```python
from build123d import *

# Parameters (mm, degrees)
F0_R      = 57.15
F3_DEPTH  = 514.096
F2_R      = 57.15
F5_DEPTH  = 104.648
F6_W      = 58.42
F6_H      = 58.42
F7_DEPTH  = 58.42
F8_W      = 58.42
F8_H      = 58.42
F9_DEPTH  = 58.42
F10_W     = 44.45
F10_H     = 44.45
F11_DEPTH = 30.48


# Not quite as in the source:
# - a feature names something its author has since deleted; it is built from what else it names


with BuildPart() as f3:
    # F0 (on Right) → F3 (new body)
    with BuildSketch(Plane.YZ):
        Circle(F0_R)
    extrude(amount=F3_DEPTH)

    # F1 (on Top) → F4 (revolve)
    with BuildSketch(Plane.XY):
        with BuildLine():
            Line((514.096, 57.15), (514.096, 0))
            Line((514.096, 0), (615.696, 0))
            Line((615.696, 0), (615.696, 44.45))
            add(Edge.make_bspline(
                [(514.096, 57.15), (530.3059150596, 55.8042351211), (558.1923144484, 54.3135523686), (580.3852464856, 48.6501982027), (594.1085406783, 43.9680323111), (608.3163207178, 44.8236773325), (615.696, 44.45)],
                knots=[0, 0, 0, 0, 0.3407026007, 0.5771106283, 0.7657914869, 1, 1, 1, 1], degree=3))
        make_face()
    revolve(axis=Axis((564.896, 0, 0), (-1, 0, 0)))

    # F2 (on Front) → F5 (join)
    with BuildSketch(Plane.XZ):
        with Locations((257.048, 0)):
            Circle(F2_R)
    extrude(amount=F5_DEPTH)

    # F6 (on face) → F7 (cut)
    with BuildSketch(Plane(origin=(0, 0, 0), x_dir=(0, -1, 0), z_dir=(-1, 0, 0))):
        Rectangle(F6_W, F6_H)
    extrude(amount=-F7_DEPTH, mode=Mode.SUBTRACT)

    # F8 (on face) → F9 (cut)
    with BuildSketch(Plane.XZ.offset(104.648)):
        with Locations((257.048, 0)):
            Rectangle(F8_W, F8_H)
    extrude(amount=-F9_DEPTH, mode=Mode.SUBTRACT)

    # F10 (on face) → F11 (cut)
    with BuildSketch(Plane.YZ.offset(615.696)):
        Rectangle(F10_W, F10_H)
    extrude(amount=-F11_DEPTH, mode=Mode.SUBTRACT)


solid = f3.part
```
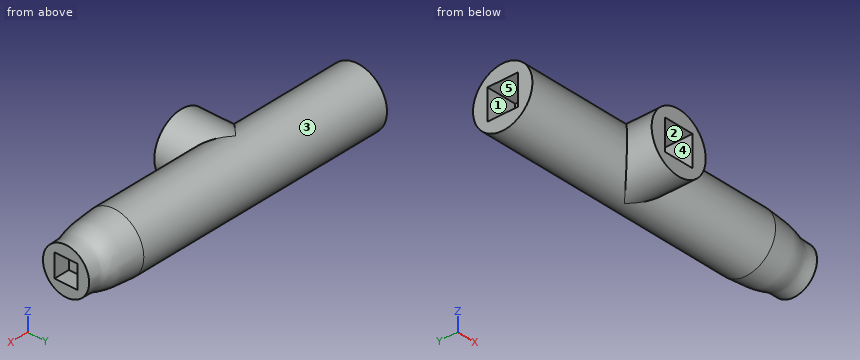
Work out the finished part from the listing and answer in its coordinate system (mm). Face numbers are marked on the shaded views. A direction names the side the tool comes from. Round coordinates to 2 decimals unless told otherwise and drop trailing zeros. Loops run counter-clockwise (first coordinate to the right, second up) from the corner with the lowest first, then second, coordinate; pieces in that order, holes last.
(1) The part is cut by section A-A, the plane x = 447. Give the vertices of the cut face in (y, z), and give its area (3 significant figures).
Computed values:
outline: circle Ø114.3 at (0, 0)
area: 10,300 mm2
(2) For the marked faces 1 and 2, determine the directions among +Z, -Z, +X, -X, +Y, -Y from which every point of the face is accessible in a straight line to the end or side of a thin tool.
Computed values:
face 1: -X
face 2: -Y
(3) Each of these flat-tipped pins is pushed along its axis until it touches: P1, Ø12, axis at x = 543.5, z = -30, coming from the -Y side; P2, Ø5, axis at x = 461, y = 32, coming from the +Z side; P3, Ø17.5, axis at y = -79, z = -8, coming from the +X side. Where does it stop, or does it pass through?
Computed values:
P1: stops at y = -49.37
P2: stops at z = 48.95
P3: stops at x = 314.2
(4) The mould has two halves that part along Y. Classify the marked faces 3, 4 and 5: pulls with the +Y half, pulls with the -Y half, needs draft (parallel to the pull), parting line crosses it, or undercut.
Computed values:
face 3: parting line crosses it
face 4: needs draft
face 5: undercut
(5) Find the intervals of material crossed by L1, parallel to X at y = 14, z = -0.5; L2, parallel to X at y = -59, z = -13; L3, parallel to X at y = 3, z = -26.5, in increasing order.
Computed values:
L1: x = 58.42 to 585.22
L2: x = 201.4 to 227.84, 286.26 to 312.7
L3: x = 58.42 to 615.7
